Work out the finished part from the listing and answer in its coordinate system (mm). Face numbers are marked on the shaded views. Give positions to 0.01 mm unless a question says otherwise; leave off trailing zeros. Order: outer loops, then holes, each group sorted by start corner. A loop starts at its lowest first (then second) coordinate and runs counter-clockwise, first axis right, second up.
```python
from build123d import *

# Parameters (mm, degrees)
F0_W     = 25.4
F0_H     = 25.4
F1_DEPTH = 72.25612
F2_R     = 7.977786
F3_DEPTH = 82.87319
F5_D     = 8.89
F5_DEPTH = 12.7
F2_W     = 25.4
F2_H     = 25.4
F2_R_2   = 10.673918
F6_DEPTH = 88.86488


with BuildPart() as f1:
    # F0 (on Right) → F1 (new body)
    with BuildSketch(Plane.YZ):
        with Locations((-33.407167, -34.459156)):
            Rectangle(F0_W, F0_H)
    extrude(amount=F1_DEPTH)

    # F2 (on face) → F3 (cut)
    with BuildSketch(Plane.YZ.offset(72.25612)):
        with Locations((-34.093928, -34.619924)):
            Circle(F2_R)
    extrude(amount=-F3_DEPTH, mode=Mode.SUBTRACT)

    # F5
    with Locations(Plane.XY.offset(-21.759156)):
        with Locations((18.0594, -33.407167), (54.18746, -33.407167)):
            Hole(F5_D / 2, depth=F5_DEPTH)

    # F2 (on face) → F6 (cut)
    with BuildSketch(Plane.YZ.offset(72.25612)):
        with Locations((-33.407167, -34.459156)):
            Rectangle(F2_W, F2_H)
        with Locations((-34.093928, -34.619924)):
            Circle(F2_R_2, mode=Mode.SUBTRACT)
    extrude(amount=-F6_DEPTH, mode=Mode.SUBTRACT)


solid = f1.part
```
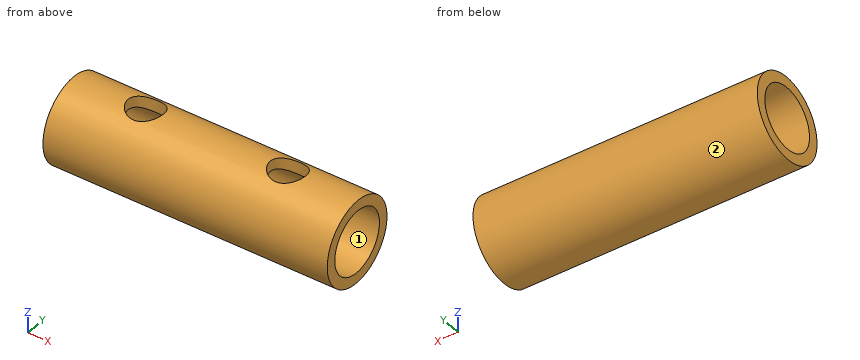
1. The part is cut by section C-C (x = 18.5). Write down the section's boundary in (y, z), then the cut area to 3 significant figures.
Findings below:
outline: (-37.83, -27.57) - (-37.83, -24.62) arc R10.67 ccw (long way) to (-28.98, -25.25) - (-28.98, -28.49) arc R7.98 cw (long way) to start
area: 133 mm2
2. The part is cut by section D-D (y = -42.75). Write down the section's boundary in (x, z).
Findings below:
outline: (0, -40.87) - (72.26, -40.87) - (72.26, -28.37) - (0, -28.37) - close
3. The part is cut by section B-B (y = -39). Write down the section's boundary in (x, z), then the cut area to 3 significant figures.
Findings below:
outline: (0, -44.1) - (72.26, -44.1) - (72.26, -40.91) - (0, -40.91) - close; (0, -28.33) - (72.26, -28.33) - (72.26, -25.14) - (0, -25.14) - close
area: 461 mm2
4. The mould has two halves that part along Z. Classify the marked faces 1 and 2: pulls with the +Z half, pulls with the -Z half, needs draft (parallel to the pull), parting line crosses it, or undercut.
Findings below:
face 1: undercut
face 2: parting line crosses it
5. Given P1, Ø1, axis at x = 13.5, z = -36, coming from the +Y side; P2, Ø3, axis at x = 19.5, y = -30.5, coming from the -Z side; P3, Ø6, axis at x = 20.5, y = -26.5, coming from the +Z side, each flat-ended and moving along its own axis, determine where each tip first touches the part or whether it passes through.
Findings below:
P1: stops at y = -23.46
P2: stops at z = -45.09
P3: stops at z = -24.99
6. The part is cut by section A-A (z = -36.5). Write down the section's boundary in (x, y).
Findings below:
outline: (0, -44.6) - (72.26, -44.6) - (72.26, -41.85) - (0, -41.85) - close; (0, -26.34) - (72.26, -26.34) - (72.26, -23.59) - (0, -23.59) - close
7. Straight lines are drawn through the part: probe 1 along Z at (x, y) = (34.5, -34.5); probe 2 along Y at (x, z) = (14, -34.25); probe 3 along Y at (x, z) = (29, -36.75). For each, find the intervals that lie inside material, in ascending order.
Findings below:
probe 1: z = -45.29 to -42.59, -26.65 to -23.95
probe 2: y = -44.76 to -42.06, -26.12 to -23.43
probe 3: y = -44.55 to -41.78, -26.41 to -23.63
